```python
from build123d import *

# Parameters (mm, degrees)
SKETCH_1_W          = 245
SKETCH_1_H          = 62
SKETCH_1_R          = 1.6
SKETCH_1_R_2        = 2.6
EXTRUDE_1_DEPTH     = 1.5
SKETCH_2_R          = 1.6
CUT_EXTRUDE_1_DEPTH = 253.740974122
SKETCH_3_OUTSIDE_W  = 297.548
SKETCH_3_OUTSIDE_H  = 114.548
CUT_EXTRUDE_2_DEPTH = 3
FILLET_1_R          = 40
FILLET_2_R          = 3
CHAMFER_1_SIZE      = 5
SKETCH_4_R          = 3.5
CUT_EXTRUDE_3_DEPTH = 252.040549253
CUT_EXTRUDE_4_REACH = 253.041
SKETCH_5_R          = 1.6


with BuildPart() as part:
    # 草图1 → 凸台-拉伸1 (new, symmetric)
    with BuildSketch(Plane.XY):
        with Locations((-122.5, -31)):
            Rectangle(SKETCH_1_W, SKETCH_1_H)
        with Locations((-112.5, -11)):
            Circle(SKETCH_1_R, mode=Mode.SUBTRACT)
        with Locations((-37.5, -11)):
            Circle(SKETCH_1_R, mode=Mode.SUBTRACT)
        with Locations(Location((-97.5, -11, 0), (0, 0, 180))):
            Circle(SKETCH_1_R, mode=Mode.SUBTRACT)
        with Locations(Location((-22.5, -11, 0), (0, 0, 180))):
            Circle(SKETCH_1_R, mode=Mode.SUBTRACT)
        with Locations((-220, -55)):
            Circle(SKETCH_1_R_2, mode=Mode.SUBTRACT)
    extrude(amount=EXTRUDE_1_DEPTH, both=True)

    # 草图2 → 切除-拉伸1 (cut, through all)
    with BuildSketch(Plane.XY.offset(1.5)):
        with Locations((-193, -10)):
            Circle(SKETCH_2_R)
        with Locations((-193, -30)):
            Circle(SKETCH_2_R)
        with Locations((-118, -20)):
            Circle(SKETCH_2_R)
    extrude(amount=-CUT_EXTRUDE_1_DEPTH, mode=Mode.SUBTRACT)

    # 草图3 outside → 切除-拉伸2 (cut)
    with BuildSketch(Plane.XY.offset(1.5)):
        with Locations((-122.5, -31)):
            Rectangle(SKETCH_3_OUTSIDE_W, SKETCH_3_OUTSIDE_H)
        Polygon((0, 0), (-244.36195996, 0), (-223, -37), (-245, -37), (-245, -62), (-173.63804004, -62), (-184.31902002, -43.5), (-74.31902002, -43.5), (-85, -25), (0, -25), align=None, mode=Mode.SUBTRACT)
    extrude(amount=-CUT_EXTRUDE_2_DEPTH, mode=Mode.SUBTRACT)

    # 圆角1
    # the kernel refuses this fillet: 40 mm, written as the material it takes off along each edge
    with BuildSketch(Plane(origin=(-245, -62, -94.202481089), x_dir=(1, 0, 0), z_dir=(0, 0, 1))) as fillet_1_piece_1:
        with BuildLine():
            CenterArc((37.080992435, 40), FILLET_1_R, 202.024312837, 67.975687163)
            Line((0, 25), (-0.741619849, 24.7))
            ThreePointArc((-0.741619849, 24.7), (-0.8, 12.5), (-0.8, 0))
            Line((-0.8, 0), (0, -0.8))
            Line((0, -0.8), (37.080992435, -0.8))
            Line((37.080992435, -0.8), (37.080992435, 0))
        make_face()
    extrude(amount=188.404962177, mode=Mode.SUBTRACT)

    # 圆角2
    fillet_2_edges = [part.edges().sort_by_distance(p)[0] for p in [
        (-85, -25, 0),
        (-74.31902002, -43.5, 0),
        (-184.31902002, -43.5, 0),
        (-173.63804004, -62, 0),
        (-245, -37, 0),
        (-223, -37, 0),
        (-244.36195996, 0, 0),
    ]]
    fillet(fillet_2_edges, radius=FILLET_2_R)

    # 倒角1
    chamfer_1_edges = [part.edges().sort_by_distance(p)[0] for p in [
        (0, -25, 0),
        (0, 0, 0),
    ]]
    chamfer(chamfer_1_edges, length=CHAMFER_1_SIZE)

    # 草图4 → 切除-拉伸3 (cut, through all)
    with BuildSketch(Plane.XY.offset(1.5)):
        with Locations((-90.5, -7.5)):
            Circle(SKETCH_4_R)
        with Locations((-79, -7.5)):
            Circle(SKETCH_4_R)
        with Locations((-67.5, -7.5)):
            Circle(SKETCH_4_R)
        with Locations((-56, -7.5)):
            Circle(SKETCH_4_R)
        with Locations((-44.5, -7.5)):
            Circle(SKETCH_4_R)
        with Locations((-79, -17.5)):
            Circle(SKETCH_4_R)
        with Locations((-67.5, -17.5)):
            Circle(SKETCH_4_R)
        with Locations((-56, -17.5)):
            Circle(SKETCH_4_R)
        with Locations((-44.5, -17.5)):
            Circle(SKETCH_4_R)
        with Locations((-90.5, -17.5)):
            Circle(SKETCH_4_R)
        Polygon((-174.543303051, -8), (-188.381197846, -8), (-172.504065444, -35.5), (-158.666170648, -35.5), align=None)
        Polygon((-152.622504486, -8), (-166.460399282, -8), (-150.583266879, -35.5), (-136.745372084, -35.5), align=None)
        Polygon((-130.701705922, -8), (-144.539600718, -8), (-128.662468315, -35.5), (-114.824573519, -35.5), align=None)
        Polygon((-214.358257627, -8), (-228.196152423, -8), (-212.31902002, -35.5), (-198.481125224, -35.5), align=None)
    extrude(amount=-CUT_EXTRUDE_3_DEPTH, mode=Mode.SUBTRACT)

    # 草图5 → 切除-拉伸4 (cut, up to next)
    with BuildSketch(Plane.XY.offset(1.5), mode=Mode.PRIVATE) as cut_extrude_4_sk1:
        with Locations((-160.004065444, -39.5)):
            Circle(SKETCH_5_R)
    cut_extrude_4_tool1 = extrude(cut_extrude_4_sk1.sketch, amount=-CUT_EXTRUDE_4_REACH, mode=Mode.PRIVATE) & part.part
    # 草图5 → 切除-拉伸4 (cut, up to next)
    with BuildSketch(Plane.XY.offset(1.5), mode=Mode.PRIVATE) as cut_extrude_4_sk2:
        with BuildLine():
            Line((-188.004065444, -37.9), (-182.004065444, -37.9))
            ThreePointArc((-182.004065444, -37.9), (-180.404065444, -39.5), (-182.004065444, -41.1))
            Line((-182.004065444, -41.1), (-188.004065444, -41.1))
            ThreePointArc((-188.004065444, -41.1), (-189.604065444, -39.5), (-188.004065444, -37.9))
        make_face()
    cut_extrude_4_tool2 = extrude(cut_extrude_4_sk2.sketch, amount=-CUT_EXTRUDE_4_REACH, mode=Mode.PRIVATE) & part.part
    add(cut_extrude_4_tool1.solids().sort_by_distance((-160.004065, -39.5, 1.5))[0], mode=Mode.SUBTRACT)
    add(cut_extrude_4_tool2.solids().sort_by_distance((-185.004065, -39.5, 1.5))[0], mode=Mode.SUBTRACT)


solid = part.part
```
Design review of the part built by this model. Coordinates are the model's own, in mm. A direction names the side the tool comes from. Coordinates: 2 decimals unless noted, no trailing zeros. Write each loop counter-clockwise with the first axis right and the second up, starting at its lowest first coordinate (ties: lowest second). Pieces come first, ordered by that corner, then holes. Notation, with made-up numbers: M -25.75,69.5 L 12.25,69.5 A33 cw 12.25,105.5 Z; hole C -20.75,59.5 d9. An arc over 180 degrees is marked long. Answer as a JSON object with one key per item and string values.
Item 1: Add section B-B, the plane z = 0. State how many separate pieces and enclosed holes the cut face has, and give its area (3 significant figures).
Outcome:
{"separate pieces": "1", "enclosed holes": "24", "area": "7,680 mm²"}
Item 2: Insertion check: pin 1 Ø8 at (x, y) = (-56, -17.5) entering from -Z; pin 2 Ø0.9 at (x, z) = (-162, 0) entering from -Y. Each pin has a flat end and moves straight along its axis. Give the tip position at first contact, or say it passes through.
Outcome:
{"pin 1": "z = -1.5", "pin 2": "y = -43.5"}
Item 3: Add section A-A, the plane x = -202.5. Give the boundary of the cut face in (y, z).
Outcome:
{"outline": "M -62,-1.5 L -35.5,-1.5 L -35.5,1.5 L -62,1.5 Z; M -28.54,-1.5 L 0,-1.5 L 0,1.5 L -28.54,1.5 Z"}
Item 4: Machinability: for faces 4 (the flat face through (-220.369, -21.558, 0.021)), 5 (the flat face through (-150, -10, -1.5)), 6 (the flat face through (-178.94, -52.82, 0.02)), 7 (the flat face through (-233.794, -18.304, 0.021)), which of the approach directions +Z, -Z, +X, -X, +Y, -Y give a long, thin tool a straight path to every point of the face, cutting with its end or side? Answer none if there is none.
Outcome:
{"face 4": "+Z, -Z", "face 5": "-Z, +X, -X, +Y, -Y", "face 6": "+Z, -Z, +X", "face 7": "+Z, -Z, -X"}
Item 5: Draft analysis for pull direction X (two halves, no side actions). For faces 1 (the cylindrical face through (-228.443, -56.333, -0.021)), 2 (the flat face through (-136.71, -21.56, 0.02)), 3 (the flat face through (-3, -23, 0)), state which applies: pulls with the +X half, pulls with the -X half, needs draft (parallel to the pull), parting line crosses it, or undercut.
Outcome:
{"face 1": "pulls with the -X half", "face 2": "undercut", "face 3": "pulls with the +X half"}
Item 6: Wall thickness on probe 1 along Y at (x, z) = (-44.5, -0.85); probe 2 along Y at (x, z) = (-90.5, 0.45); probe 3 along Y at (x, z) = (-22.5, -0.6): over which ranges is each line inside the solid? List them lowest first.
Outcome:
{"probe 1": "-25 to -21, -14 to -11, -4 to 0", "probe 2": "-43.5 to -21, -14 to -11, -4 to 0", "probe 3": "-25 to -12.6, -9.4 to 0"}
